from build123d import *

# Parameters (mm, degrees)
F0_R          = 2.6
F1_DEPTH      = 6
F2_R          = 5
F3_DEPTH      = 5
F3_DEPTH_BACK = 2
F4_R          = 1.6
F5_DEPTH      = 7.001


with BuildPart() as f1:
    # F0 (on Top) → F1 (new body)
    with BuildSketch(Plane.XY):
        with BuildLine():
            Line((-15, -5), (15, -5))
            ThreePointArc((15, -5), (18.535534, -3.535534), (20, 0))
            ThreePointArc((20, 0), (18.535534, 3.535534), (15, 5))
            Line((15, 5), (-15, 5))
            ThreePointArc((-15, 5), (-18.535534, 3.535534), (-20, 0))
            ThreePointArc((-20, 0), (-18.535534, -3.535534), (-15, -5))
        make_face()
        with Locations((-15, 0)):
            Circle(F0_R, mode=Mode.SUBTRACT)
        with Locations((15, 0)):
            Circle(F0_R, mode=Mode.SUBTRACT)
    extrude(amount=F1_DEPTH)

    # F2 (on Front) → F3 (join, two sides)
    with BuildSketch(Plane.XZ) as f3_sk:
        with BuildLine():
            Line((10, 6), (10, 16))
            ThreePointArc((10, 16), (0, 26), (-10, 16))
            Line((-10, 16), (-10, 6))
            Line((-10, 6), (10, 6))
        make_face()
        with Locations((0, 16)):
            Circle(F2_R, mode=Mode.SUBTRACT)
    extrude(amount=F3_DEPTH)
    extrude(f3_sk.sketch, amount=-F3_DEPTH_BACK)

    # F4 (on face) → F5 (cut, through all)
    with BuildSketch(Plane(origin=(0, 2, 0), x_dir=(-1, 0, 0), z_dir=(0, 1, 0))):
        with Locations((0, 24)):
            Circle(F4_R)
        with Locations((8, 16)):
            Circle(F4_R)
        with Locations((0, 8)):
            Circle(F4_R)
        with Locations((-8, 16)):
            Circle(F4_R)
    extrude(amount=-F5_DEPTH, mode=Mode.SUBTRACT)


solid = f1.part
Can you work these out from the model? Positions are in its coordinate system, mm. A direction names the side the tool comes from. Give positions to 0.01 mm unless a question says otherwise; leave off trailing zeros. Loops run counter-clockwise (first coordinate to the right, second up) from the corner with the lowest first, then second, coordinate; pieces in that order, holes last. Notation, with made-up numbers: (57, 24.25) - (71, 24.25) arc R9 ccw to (71, 34.25) - close; hole circle Ø4 at (74.25, -21.5). An arc over 180 degrees is marked (long way). One line per item, written item: value.
(1) I need wall thicknesses on line 1 along Z through (x, y) = (0, 1.65); line 2 along Y through (x, z) = (15, 4.1); line 3 along Z through (x, y) = (8, -2.25). Which ranges of each line are inside material? Lowest first, please.
Verdict:
line 1: 0 to 6.4, 9.6 to 11, 21 to 22.4, 25.6 to 26
line 2: -5 to -2.6, 2.6 to 5
line 3: 0 to 14.4, 17.6 to 22
(2) If we mould it in two halves opening along Z, with no side actions, what happens to faces 4 (the face through (0, -5, 10)), 5 (the face through (-0.3, 2.3, 6)), 6 (the face through (8.208, -1.451, 17.586))? For each: released by +Z, released by -Z, zero draft, split by the parting line, or undercut.
Verdict:
face 4: zero draft
face 5: released by +Z
face 6: undercut
(3) On a 3-axis mill with a long thin cutter (end or side, diameter ignored), from which of +Z, -Z, +X, -X, +Y, -Y can I reach the whole of each face in a straight line? I mean faces 1 (the face through (-5, 2, 14)), 2 (the face through (10, -2, 11)), 3 (the face through (-10, -2, 11)). Say none if no direction works.
Verdict:
face 1: +Z, +X, -X, +Y
face 2: +Z, +X, +Y, -Y
face 3: +Z, -X, +Y, -Y
(4) If we section it at C-C, the plane z = 2: List the corners of the cut face in (x, y) for me.
Verdict:
outline: (-15, -5) - (15, -5) arc R5 ccw to (15, 5) - (-15, 5) arc R5 ccw to start; hole circle Ø5.2 at (-15, 0); hole circle Ø5.2 at (15, 0)
(5) If we section it at B-B, the plane x = -8: List the corners of the cut face in (y, z) for me.
Verdict:
outline: (-5, 0) - (5, 0) - (5, 6) - (2, 6) - (2, 14.4) - (-5, 14.4) - close; (-5, 17.6) - (2, 17.6) - (2, 22) - (-5, 22) - close
(6) If we section it at A-A, the plane x = 0: List the corners of the cut face in (y, z) for me, plus the area to 3 significant figures.
Verdict:
outline: (-5, 0) - (5, 0) - (5, 6) - (2, 6) - (2, 6.4) - (-5, 6.4) - close; (-5, 9.6) - (2, 9.6) - (2, 11) - (-5, 11) - close; (-5, 21) - (2, 21) - (2, 22.4) - (-5, 22.4) - close; (-5, 25.6) - (2, 25.6) - (2, 26) - (-5, 26) - close
area: 85.2 mm^2
(7) I'm going to push flat-ended pins straight in: pin 1 (6 mm diameter, centred on x = -15, y = 0, fed in from +Z); pin 2 (2 mm diameter, centred on y = -0.5, z = 3, fed in from +X); pin 3 (3.5 mm diameter, centred on x = 0, z = 24, fed in from +Y); pin 4 (1.9 mm diameter, centred on x = -8, z = 16, fed in from -Y). Where does each tip first touch, or does it pass through?
Verdict:
pin 1: z = 6
pin 2: x = 20
pin 3: y = 2
pin 4: through
(8) If we section it at D-D, the plane y = 0.5: List the corners of the cut face in (x, z) for me.
Verdict:
outline: (-19.97, 0) - (-17.55, 0) - (-17.55, 6) - (-19.97, 6) - close; (-12.45, 0) - (12.45, 0) - (12.45, 6) - (10, 6) - (10, 16) arc R10 ccw to (-10, 16) - (-10, 6) - (-12.45, 6) - close; (17.55, 0) - (19.97, 0) - (19.97, 6) - (17.55, 6) - close; hole circle Ø3.2 at (-8, 16); hole circle Ø10 at (0, 16); hole circle Ø3.2 at (0, 8); hole circle Ø3.2 at (0, 24); hole circle Ø3.2 at (8, 16)
